from build123d import *

# Parameters (mm, degrees)
SKETCH1_W           = 58
SKETCH1_H           = 37
SKETCH1_R           = 2.25
SKETCH1_W_2         = 42
SKETCH1_H_2         = 21
BOSS_EXTRUDE1_DEPTH = 5
SKETCH2_W           = 42
SKETCH2_H           = 8
BOSS_EXTRUDE2_DEPTH = 17
SKETCH3_W           = 42
SKETCH3_H           = 42
BOSS_EXTRUDE3_DEPTH = 5
FILLET1_R           = 5
FILLET2_R           = 5
FILLET3_R           = 5
FILLET4_R           = 5
FILLET5_R           = 5
FILLET6_R           = 5
FILLET7_R           = 5


with BuildPart() as part:
    # Sketch1 → Boss-Extrude1 (new body)
    with BuildSketch(Plane.XY):
        Rectangle(SKETCH1_W, SKETCH1_H)
        with Locations((-24.5, 5)):
            Circle(SKETCH1_R, mode=Mode.SUBTRACT)
        with Locations((-24.5, -5)):
            Circle(SKETCH1_R, mode=Mode.SUBTRACT)
        with Locations(Location((24.5, 5, 0), (0, 0, 180))):
            Circle(SKETCH1_R, mode=Mode.SUBTRACT)
        with Locations(Location((24.5, -5, 0), (0, 0, 180))):
            Circle(SKETCH1_R, mode=Mode.SUBTRACT)
        Rectangle(SKETCH1_W_2, SKETCH1_H_2, mode=Mode.SUBTRACT)
    extrude(amount=BOSS_EXTRUDE1_DEPTH)

    # Sketch2 → Boss-Extrude2 (add)
    with BuildSketch(Plane.XY.offset(5)):
        with Locations((0, 14.5)):
            Rectangle(SKETCH2_W, SKETCH2_H)
        with Locations((0, -14.5)):
            Rectangle(SKETCH2_W, SKETCH2_H)
    extrude(amount=BOSS_EXTRUDE2_DEPTH)

    # Sketch3 → Boss-Extrude3 (add)
    with BuildSketch(Plane.XY.offset(22)):
        with Locations((0, -31.5)):
            Rectangle(SKETCH3_W, SKETCH3_H)
        with Locations((0, 31.5)):
            Rectangle(SKETCH3_W, SKETCH3_H)
    extrude(amount=BOSS_EXTRUDE3_DEPTH)

    # Fillet1
    fillet1_edges = [part.edges().sort_by_distance(p)[0] for p in [
        (0, 18.5, 22),
    ]]
    fillet(fillet1_edges, radius=FILLET1_R)

    # Fillet2
    fillet2_edges = [part.edges().sort_by_distance(p)[0] for p in [
        (0, -18.5, 22),
    ]]
    fillet(fillet2_edges, radius=FILLET2_R)

    # Fillet3
    fillet3_edges = [part.edges().sort_by_distance(p)[0] for p in [
        (0, 52.5, 22),
    ]]
    fillet(fillet3_edges, radius=FILLET3_R - 0.0001)  # a hair under: the kernel refuses the full size

    # Fillet4
    fillet4_edges = [part.edges().sort_by_distance(p)[0] for p in [
        (0, -52.5, 22),
    ]]
    fillet(fillet4_edges, radius=FILLET4_R - 0.0001)  # a hair under: the kernel refuses the full size

    # Fillet5
    fillet5_edges = [part.edges().sort_by_distance(p)[0] for p in [
        (-21, 51.035563195, 23.464436805),
        (-21, 18.5, 11),
        (-21, 19.964466094, 20.535533906),
        (21, 18.5, 11),
        (21, 19.964466094, 20.535533906),
        (21, 51.035563195, 23.464436805),
        (-21, 35.50005, 22),
        (21, 35.50005, 22),
    ]]
    fillet(fillet5_edges, radius=FILLET5_R - 0.0001)  # a hair under: the kernel refuses the full size

    # Fillet6
    fillet6_edges = [part.edges().sort_by_distance(p)[0] for p in [
        (-21, -35.50005, 22),
        (21, -18.5, 11),
        (-21, -18.5, 11),
        (21, -19.964466094, 20.535533906),
        (-21, -19.964466094, 20.535533906),
        (21, -35.50005, 22),
        (21, -51.035563195, 23.464436805),
        (-21, -51.035563195, 23.464436805),
    ]]
    fillet(fillet6_edges, radius=FILLET6_R - 0.0001)  # a hair under: the kernel refuses the full size

    # Fillet7
    fillet7_edges = [part.edges().sort_by_distance(p)[0] for p in [
        (-29, 18.5, 2.5),
        (-29, -18.5, 2.5),
        (29, -18.5, 2.5),
        (29, 18.5, 2.5),
    ]]
    fillet(fillet7_edges, radius=FILLET7_R)


solid = part.part
Geometry: final body of the model. Coordinates: model frame, mm. A direction names the side the tool comes from. Give positions to 0.01 mm unless a question says otherwise; leave off trailing zeros. Loops run counter-clockwise (first coordinate to the right, second up) from the corner with the lowest first, then second, coordinate; pieces in that order, holes last. Notation, with made-up numbers: M 63.25,53.25 L 120.25,53.25 A22 cw 120.25,73.25 Z; hole C 17,33.5 d9. An arc over 180 degrees is marked long. Put each result on its own line as item: value. Start each with the question number.
1) Contact query for flat-ended pins moving along their axis: pin 1 (5 mm diameter, centred on x = -16.5, z = 16, fed in from -Y); pin 2 (1.5 mm diameter, centred on y = 12.5, z = 6, fed in from +X); pin 3 (3.5 mm diameter, centred on x = 24.5, y = 5, fed in from +Z); pin 4 (12 mm diameter, centred on x = 4, y = 30, fed in from -Z). Output: stop coordinate, or through.
2) Cut plane A-A (y = 5). Output: boundary loops of the cut face in (x, z), then the cut area to 3 significant figures.
3) Ray query, line 1 along Y through (x, z) = (-24.5, 2.45); line 2 along Y through (x, z) = (-11, 13.75); line 3 along Z through (x, y) = (-8, -41.5). Return the intervals inside material, ascending.
4) Cut plane B-B (z = 2). Output: boundary loops of the cut face in (x, y).
5) Cut plane D-D (z = 9.5). Output: boundary loops of the cut face in (x, y).
6) Pull-direction query (X, two-part tool) for faces 6 (the flat face through (-24, 0, 5)), 7 (the cylindrical face through (22.354, 4.324, 2.465)), 8 (the flat face through (21, -13, 18)); classes: pulls with the +X half, pulls with the -X half, needs draft (parallel to the pull), parting line crosses it, or undercut.
7) Access query for faces 1 (the cylindrical face through (19, 36, 23)), 2 (the flat face through (21, 0, 2)), 3 (the flat face through (-21, -13, 18)), 4 (the cylindrical face through (19.5, 17.07, 11.08)), 5 (the flat face through (0, 36, 22)). Directions: +Z, -Z, +X, -X, +Y, -Y. A direction counts if a zero-diameter tool reaches every point of the face in a straight line with its end or side. Return the directions, or none.
Verdict:
1. pin 1: y = -18.72
1. pin 2: x = 21
1. pin 3: through
1. pin 4: z = 22
2. outline: M -29,0 L -26.75,0 L -26.75,5 L -29,5 Z; M -22.25,0 L -21,0 L -21,5 L -22.25,5 Z; M 21,0 L 22.25,0 L 22.25,5 L 21,5 Z; M 26.75,0 L 29,0 L 29,5 L 26.75,5 Z
2. area: 35.0 mm2
3. line 1: -18.47 to -7.25, -2.75 to 2.75, 7.25 to 18.47
3. line 2: -18.5 to -10.5, 10.5 to 18.5
3. line 3: 22 to 27
4. outline: M -29,-13.5 A5 ccw -24,-18.5 L 24,-18.5 A5 ccw 29,-13.5 L 29,13.5 A5 ccw 24,18.5 L -24,18.5 A5 ccw -29,13.5 Z; hole C -24.5,-5 d4.5; hole C -24.5,5 d4.5; hole M -21,-10.5 L 21,-10.5 L 21,10.5 L -21,10.5 Z; hole C 24.5,-5 d4.5; hole C 24.5,5 d4.5
5. outline: M -21,-13.5 A5 ccw -16,-18.5 L 16,-18.5 A5 ccw 21,-13.5 L 21,-10.5 L -21,-10.5 Z; M -21,10.5 L 21,10.5 L 21,13.5 A5 ccw 16,18.5 L -16,18.5 A5 ccw -21,13.5 Z
6. face 6: needs draft
6. face 7: undercut
6. face 8: pulls with the +X half
7. face 1: -Z, +X, +Y
7. face 2: +Z, -Z
7. face 3: +Z, -X, +Y, -Y
7. face 4: +X, +Y
7. face 5: -Z, +X, -X, +Y
